Could you check a few things on this model? Use its own coordinates, in mm. Round coordinates to 2 decimals unless told otherwise and drop trailing zeros. Write each loop counter-clockwise with the first axis right and the second up, starting at its lowest first coordinate (ties: lowest second). Pieces come first, ordered by that corner, then holes.
```python
from build123d import *

# Parameters (mm, degrees)
BOARD_DEPTH                        = 1.59
F_1_0_228_DIAMETER_HOLE1_OUTLINE_R = 0.35
F_1_0_228_DIAMETER_HOLE1_DEPTH     = 1.59
SKETCH4_R                          = 1.1
CUT_EXTRUDE1_DEPTH                 = 106.554608126


# Read off the part's stored shape, not the designer's step: #1 (0.228) Diameter Hole1
with BuildPart() as part:
    # Sketch1 → Board (new body)
    with BuildSketch(Plane.XY):
        with BuildLine():
            Line((27.45799, 93.788), (27.45799, 94.5))
            Line((27.45799, 94.5), (22.99997, 94.5))
            Line((22.99997, 94.5), (22.99997, 85.5))
            Line((22.99997, 85.5), (27.45799, 85.49998))
            Line((27.45799, 85.49998), (27.45799, 86.18801))
            ThreePointArc((27.45799, 86.18801), (28.00799, 86.73801), (28.55799, 86.18801))
            Line((28.55799, 86.18801), (28.55799, 85.49998))
            Line((28.55799, 85.49998), (32.49999, 85.49998))
            ThreePointArc((32.49999, 85.49998), (33.49997, 86.49998), (34.49997, 85.5))
            Line((34.49997, 85.5), (42.49997, 85.5))
            ThreePointArc((42.49997, 85.5), (46.999970177, 90), (42.49997, 94.5))
            Line((42.49997, 94.5), (34.49997, 94.5))
            ThreePointArc((34.49997, 94.5), (33.49997, 93.5), (32.49997, 94.5))
            Line((32.49997, 94.5), (28.55799, 94.5))
            Line((28.55799, 94.5), (28.55799, 93.788))
            ThreePointArc((28.55799, 93.788), (28.00799, 93.238), (27.45799, 93.788))
        make_face()
    extrude(amount=BOARD_DEPTH)

    # #1 (0.228) Diameter Hole1 outline → #1 (0.228) Diameter Hole1 (cut)
    with BuildSketch(Plane.XY):
        with Locations((29.85799, 92.238)):
            Circle(F_1_0_228_DIAMETER_HOLE1_OUTLINE_R)
        with Locations((26.15799, 90.738)):
            Circle(F_1_0_228_DIAMETER_HOLE1_OUTLINE_R)
        with Locations((29.85799, 89.238)):
            Circle(F_1_0_228_DIAMETER_HOLE1_OUTLINE_R)
        with Locations((26.15799, 87.738)):
            Circle(F_1_0_228_DIAMETER_HOLE1_OUTLINE_R)
    extrude(amount=F_1_0_228_DIAMETER_HOLE1_DEPTH, mode=Mode.SUBTRACT)

    # Sketch4 → Cut-Extrude1 (cut, through all)
    with BuildSketch(Plane.XY.offset(1.59)):
        with Locations((33.49997, 90)):
            Circle(SKETCH4_R)
    extrude(amount=-CUT_EXTRUDE1_DEPTH, mode=Mode.SUBTRACT)


solid = part.part
```
Q1. We'd pull the mould along X, two halves only. Please class faces 1 (the flat face through (31, 94.5, 1)), 2 (the cylindrical face through (33.5, 86.5, 0.8)), 3 (the cylindrical face through (47, 90, 1)): pulls with the +X half, pulls with the -X half, needs draft (parallel to the pull), parting line crosses it, or undercut.
Q2. Imagine slicing it at C-C, the plane z = 1.15. Write out the boundary of the cut face in (x, y).
Q3. Imagine slicing it at B-B, the plane x = 33. Write out the boundary of the cut face in (y, z), then the cut area to 3 significant figures.
Q4. I'm going to push flat-ended pins straight in: pin 1 Ø0.8 at (y, z) = (94, 1) entering from +X; pin 2 Ø1.3 at (x, y) = (33.5, 90) entering from -Z. Where does each tip first touch, or does it pass through?
Q5. Imagine slicing it at A-A, the plane y = 90. Write out the boundary of the cut face in (x, z).
Q6. If I drill on L1, parallel to Y at x = 29.75, z = 1.2; L2, parallel to X at y = 89, z = 0.4; L3, parallel to X at y = 90, z = 1.5, over which ranges is the centre line in solid material (lowest first)?
Results found:
1. face 1: needs draft
1. face 2: undercut
1. face 3: pulls with the +X half
2. outline: (23, 85.5) - (27.46, 85.5) - (27.46, 86.19) arc R0.55 cw to (28.56, 86.19) - (28.56, 85.5) - (32.5, 85.5) arc R1 cw to (34.5, 85.5) - (42.5, 85.5) arc R4.5 ccw to (42.5, 94.5) - (34.5, 94.5) arc R1 cw to (32.5, 94.5) - (28.56, 94.5) - (28.56, 93.79) arc R0.55 cw to (27.46, 93.79) - (27.46, 94.5) - (23, 94.5) - close; hole circle Ø0.7 at (26.16, 87.74); hole circle Ø0.7 at (26.16, 90.74); hole circle Ø0.7 at (29.86, 89.24); hole circle Ø0.7 at (29.86, 92.24); hole circle Ø2.2 at (33.5, 90)
3. outline: (86.37, 0) - (89.02, 0) - (89.02, 1.59) - (86.37, 1.59) - close; (90.98, 0) - (93.63, 0) - (93.63, 1.59) - (90.98, 1.59) - close
3. area: 8.44 mm2
4. pin 1: stops at x = 45.2
4. pin 2: passes through
5. outline: (23, 0) - (32.4, 0) - (32.4, 1.59) - (23, 1.59) - close; (34.6, 0) - (47, 0) - (47, 1.59) - (34.6, 1.59) - close
6. L1: y = 85.5 to 88.91, 89.57 to 91.91, 92.57 to 94.5
6. L2: x = 23 to 29.6, 30.11 to 33.04, 33.96 to 46.89
6. L3: x = 23 to 32.4, 34.6 to 47
